Here's how the part is built. I have some questions about the finished solid (model axes, mm). Face numbers are marked on the shaded views. A direction names the side the tool comes from. Round coordinates to 2 decimals unless told otherwise and drop trailing zeros. Loops run counter-clockwise (first coordinate to the right, second up) from the corner with the lowest first, then second, coordinate; pieces in that order, holes last. Notation, with made-up numbers: (-18.5, -30.5) -> (0.5, -30.5) arc R22 ccw to (0.5, 4.5) -> close; hole circle Ø1 at (80, -17.5). An arc over 180 degrees is marked (long way). One line per item, written item: value. Start each with the question number.
```python
from build123d import *

# Parameters (mm, degrees)
SKETCH_W        = 32
SKETCH_H        = 18
SKETCH_R        = 1.6
PAD_DEPTH       = 12
SKETCH001_W     = 15
SKETCH001_H     = 6
POCKET_DEPTH    = 32.001
SKETCH002_R     = 1.5
POCKET001_DEPTH = 18.001


with BuildPart() as part:
    # Sketch → Pad (new body)
    with BuildSketch(Plane.XY):
        with Locations((16, 9)):
            Rectangle(SKETCH_W, SKETCH_H)
        with Locations((7, 13)):
            Circle(SKETCH_R, mode=Mode.SUBTRACT)
        with Locations((25, 13)):
            Circle(SKETCH_R, mode=Mode.SUBTRACT)
    extrude(amount=PAD_DEPTH)

    # Sketch001 → Pocket (cut, through all)
    with BuildSketch(Plane.YZ.offset(32)):
        with Locations((10.5, 6)):
            Rectangle(SKETCH001_W, SKETCH001_H)
    extrude(amount=-POCKET_DEPTH, mode=Mode.SUBTRACT)

    # Sketch002 → Pocket001 (cut, through all)
    with BuildSketch(Plane.XZ):
        with Locations((6.4, 6)):
            Circle(SKETCH002_R)
        with Locations((12.8, 6)):
            Circle(SKETCH002_R)
        with Locations((19.2, 6)):
            Circle(SKETCH002_R)
        with Locations((25.6, 6)):
            Circle(SKETCH002_R)
    extrude(amount=-POCKET001_DEPTH, mode=Mode.SUBTRACT)


solid = part.part
```
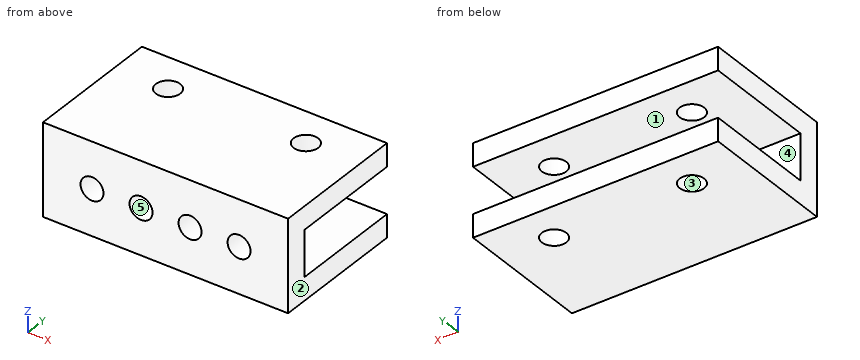
Q1. I want a section at C-C on x = 12.8. Please give me the cut outline in (y, z), plus the area to 3 significant figures.
Q2. I want a section at D-D on y = 15.75. Please give me the cut outline in (x, z), plus the area to 3 significant figures.
Q3. I want a section at A-A on z = 6. Please give me the cut outline in (x, y), plus the area to 3 significant figures.
Q4. Will these pins go through, and if not, where does the flat tip stop? P1, Ø3.5, axis at x = 19.2, z = 6, coming from the +Y side; P2, Ø3.5, axis at x = 25, y = 13, coming from the -Z side; P3, Ø3, axis at x = 7, y = 13, coming from the +Z side.
Q5. I want a section at B-B on y = 1.25. Please give me the cut outline in (x, z), plus the area to 3 significant figures.
Q6. Which directions (+Z, -Z, +X, -X, +Y, -Y) give clear straight access to the entire face, cutting with the end or side of a thin tool? Please do the marked faces 4 and 5.
Q7. If we mould it in two halves opening along X, with no side actions, what happens to the marked faces 1, 2 and 3? For each: released by +X, released by -X, zero draft, split by the parting line, or undercut.
Q8. If I drill on line 1 along X through (y, z) = (13, 11.3); line 2 along Z through (x, y) = (26.5, 5); line 3 along Y through (x, z) = (25, 1.85), over which ranges is the centre line in solid material (lowest first)?
Answers below:
1. outline: (0, 0) -> (18, 0) -> (18, 3) -> (3, 3) -> (3, 4.5) -> (0, 4.5) -> close; (0, 7.5) -> (3, 7.5) -> (3, 9) -> (18, 9) -> (18, 12) -> (0, 12) -> close
1. area: 117 mm^2
2. outline: (0, 0) -> (32, 0) -> (32, 3) -> (0, 3) -> close; (0, 9) -> (32, 9) -> (32, 12) -> (0, 12) -> close
2. area: 192 mm^2
3. outline: (0, 0) -> (4.9, 0) -> (4.9, 3) -> (0, 3) -> close; (7.9, 0) -> (11.3, 0) -> (11.3, 3) -> (7.9, 3) -> close; (14.3, 0) -> (17.7, 0) -> (17.7, 3) -> (14.3, 3) -> close; (20.7, 0) -> (24.1, 0) -> (24.1, 3) -> (20.7, 3) -> close; (27.1, 0) -> (32, 0) -> (32, 3) -> (27.1, 3) -> close
3. area: 60.0 mm^2
4. P1: stops at y = 3
4. P2: stops at z = 0
4. P3: passes through
5. outline: (0, 0) -> (32, 0) -> (32, 12) -> (0, 12) -> close; hole circle Ø3 at (6.4, 6); hole circle Ø3 at (12.8, 6); hole circle Ø3 at (19.2, 6); hole circle Ø3 at (25.6, 6)
5. area: 356 mm^2
6. face 4: +X, -X, +Y
6. face 5: +Y, -Y
7. face 1: zero draft
7. face 2: released by +X
7. face 3: undercut
8. line 1: x = 0 to 5.4, 8.6 to 23.4, 26.6 to 32
8. line 2: z = 0 to 3, 9 to 12
8. line 3: y = 0 to 11.4, 14.6 to 18
